Part model, mm, in its own coordinate system. Face numbers are marked on the shaded views. A direction names the side the tool comes from. Give positions to 0.01 mm unless a question says otherwise; leave off trailing zeros. Order: outer loops, then holes, each group sorted by start corner. A loop starts at its lowest first (then second) coordinate and runs counter-clockwise, first axis right, second up. Notation, with made-up numbers: (66.5, -16) - (100.5, -16) arc R26 ccw to (100.5, 19) - close; hole circle Ø4 at (31, -24.5). An arc over 180 degrees is marked (long way). Use a Markdown table: item, result. Add a question column.
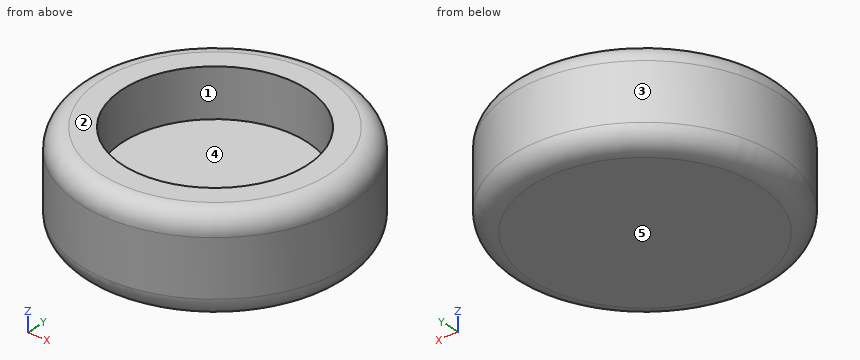
from build123d import *

# Parameters (mm, degrees)
ESQUISSE1_R             = 33.5
BOSS_EXTRU_1_DEPTH      = 24
CONG_1_R                = 5
CONG_2_R                = 5
ESQUISSE2_R             = 23
ENL_V_MAT_EXTRU_1_DEPTH = 12


with BuildPart() as part:
    # Esquisse1 → Boss.-Extru.1 (new body)
    with BuildSketch(Plane.XY):
        Circle(ESQUISSE1_R)
    extrude(amount=BOSS_EXTRU_1_DEPTH)

    # Congé1
    cong_1_edges = [part.edges().sort_by_distance(p)[0] for p in [
        (-33.5, 0, 24),
    ]]
    fillet(cong_1_edges, radius=CONG_1_R)

    # Congé2
    cong_2_edges = [part.edges().sort_by_distance(p)[0] for p in [
        (-33.5, 0, 0),
    ]]
    fillet(cong_2_edges, radius=CONG_2_R)

    # Esquisse2 → Enlèv. mat.-Extru.1 (cut)
    with BuildSketch(Plane.XY.offset(24)):
        Circle(ESQUISSE2_R)
    extrude(amount=-ENL_V_MAT_EXTRU_1_DEPTH, mode=Mode.SUBTRACT)


solid = part.part
1. Tool access for the marked faces 4 and 5: list every direction of +Z, -Z, +X, -X, +Y, -Y with a clear straight run to the whole face (end or side of a thin tool).
2. Cut at C-C (z = 14.5). Write the cut outline in (x, y), plus the area to 3 significant figures.
3. Pin check, flat tips, straight feed: P1, Ø10, axis at x = 22.5, z = 21, coming from the -Y side; P2, Ø6, axis at y = -7.5, z = 6.5, coming from the -X side; P3, Ø3, axis at x = 10, y = 5.5, coming from the -Z side; P4, Ø4, axis at y = -20, z = 3.5, coming from the -X side. Stop position of each tip, or through.
4. Cut at A-A (x = 0). Write the cut outline in (y, z), plus the area to 3 significant figures.
5. Drill centre lines: probe 1 along Y at (x, z) = (0, 15.5); probe 2 along Z at (x, y) = (-20, 6); probe 3 along Y at (x, z) = (-3.5, 21.25). Where is each one in solid material? Low to high. Write a range as [from, to].
6. Mould opens along X. For the marked faces 1, 2 and 3 say: released by +X, released by -X, zero draft, split by the parting line, or undercut.
7. Cut at D-D (z = 22.5). Write the cut outline in (x, y).
Responses:
| question | item | result |
|---|---|---|
| 1 | face 4 | +Z |
| 1 | face 5 | -Z, +X, -X, +Y, -Y |
| 2 | outline | circle Ø67 at (0, 0); hole circle Ø46 at (0, 0) |
| 2 | area | 1,860 mm² |
| 3 | P1 | stops at y = -28.4 |
| 3 | P2 | stops at x = -33.2 |
| 3 | P3 | stops at z = 0 |
| 3 | P4 | stops at x = -28.1 |
| 4 | outline | (-33.5, 5) arc R5 ccw to (-28.5, 0) - (28.5, 0) arc R5 ccw to (33.5, 5) - (33.5, 19) arc R5 ccw to (28.5, 24) - (23, 24) - (23, 12) - (-23, 12) - (-23, 24) - (-28.5, 24) arc R5 ccw to (-33.5, 19) - close |
| 4 | area | 1,030 mm² |
| 5 | probe 1 | y = [-33.5, -23], [23, 33.5] |
| 5 | probe 2 | z = [0, 12] |
| 5 | probe 3 | y = [-32.78, -22.73], [22.73, 32.78] |
| 6 | face 1 | undercut |
| 6 | face 2 | zero draft |
| 6 | face 3 | split by the parting line |
| 7 | outline | circle Ø64.14 at (0, 0); hole circle Ø46 at (0, 0) |
